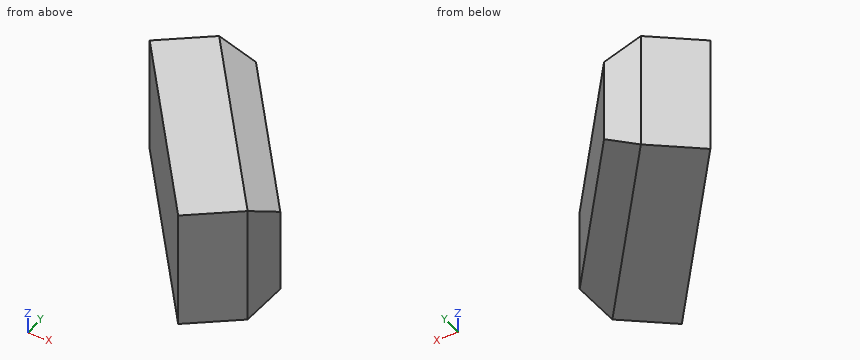
from build123d import *

# Parameters (mm, degrees)
SKETCH2_W             = 40
SKETCH2_H             = 80
BOSS_EXTRUDE1_DEPTH   = 30
CHAMFER1_SIZE         = 10
CHAMFER1_SIZE2        = 5.773502692
CHAMFER1_PART_2_SIZE  = 10
CHAMFER1_PART_2_SIZE2 = 5.773502692
CHAMFER1_PART_3_SIZE  = 10
CHAMFER1_PART_3_SIZE2 = 5.773502692
CHAMFER1_PART_4_SIZE  = 10
CHAMFER1_PART_4_SIZE2 = 5.773502692


with BuildPart() as part:
    # Sketch2 → Boss-Extrude1 (new body)
    with BuildSketch(Plane(origin=(0, 0, 0), x_dir=(0, 0, -1), z_dir=(0.788010754, 0.615661475, 0))):
        with Locations((20, 40)):
            Rectangle(SKETCH2_W, SKETCH2_H)
    extrude(amount=BOSS_EXTRUDE1_DEPTH)

    # Chamfer1
    chamfer1_edges = [part.edges().sort_by_distance(p)[0] for p in [
        (-0.986136405, 49.990274404, -40),
    ]]
    chamfer1_side = [part.faces().sort_by_distance(p)[0] for p in [
        (-12.806297709, 40.755352274, -40),
    ]]
    chamfer(chamfer1_edges, length=CHAMFER1_SIZE, length2=CHAMFER1_SIZE2, reference=chamfer1_side[0])

    # Chamfer1 part 2
    chamfer1_part_2_edges = [part.edges().sort_by_distance(p)[0] for p in [
        (-25.612595418, 81.510704548, -20),
    ]]
    chamfer1_part_2_side = [part.faces().sort_by_distance(p)[0] for p in [
        (-37.432756722, 72.275782418, -20),
    ]]
    chamfer(chamfer1_part_2_edges, length=CHAMFER1_PART_2_SIZE, length2=CHAMFER1_PART_2_SIZE2, reference=chamfer1_part_2_side[0])

    # Chamfer1 part 3
    chamfer1_part_3_edges = [part.edges().sort_by_distance(p)[0] for p in [
        (-0.986136405, 49.990274404, 0),
    ]]
    chamfer1_part_3_side = [part.faces().sort_by_distance(p)[0] for p in [
        (-12.806297709, 40.755352274, 0),
    ]]
    chamfer(chamfer1_part_3_edges, length=CHAMFER1_PART_3_SIZE, length2=CHAMFER1_PART_3_SIZE2, reference=chamfer1_part_3_side[0])

    # Chamfer1 part 4
    chamfer1_part_4_edges = [part.edges().sort_by_distance(p)[0] for p in [
        (23.640322608, 18.46984426, -20),
    ]]
    chamfer1_part_4_side = [part.faces().sort_by_distance(p)[0] for p in [
        (11.820161304, 9.23492213, -20),
    ]]
    chamfer(chamfer1_part_4_edges, length=CHAMFER1_PART_4_SIZE, length2=CHAMFER1_PART_4_SIZE2, reference=chamfer1_part_4_side[0])


solid = part.part
Verification items for the finished model (mm, model axes). Coordinates: 2 decimals unless noted, no trailing zeros. Order: outer loops, then holes, each group sorted by start corner. A loop starts at its lowest first (then second) coordinate and runs counter-clockwise, first axis right, second up.
1. Sectioned sample at A-A, the plane z = -13. Record the cut outline in (x, y).
Results found:
outline: (-49.25, 63.04) - (0, 0) - (15.76, 12.31) - (20.09, 23.02) - (-22.06, 76.96) - (-33.49, 75.35) - close
2. Sectioned sample at B-B, the plane x = 6.5. Record the cut outline in (y, z).
Results found:
outline: (5.08, -40) - (24.17, -40) - (40.41, -34.23) - (40.41, -5.77) - (24.17, 0) - (5.08, 0) - close
3. Sectioned sample at C-C, the plane y = 11. Record the cut outline in (x, z), and give its area (3 significant figures).
Results found:
outline: (-8.59, -40) - (14.08, -40) - (14.08, 0) - (-8.59, 0) - close
area: 907 mm2
4. Sectioned sample at D-D, the plane x = -39.5. Record the cut outline in (y, z).
Results found:
outline: (50.56, -40) - (70.66, -40) - (70.66, 0) - (50.56, 0) - close
5. Scan lines: line 1 (Y direction, x = -44.5, z = -10); line 2 (Y direction, x = -30, z = -15.5); line 3 (X direction, y = 22, z = -29.5). Record each from-to range of solid material in increasing order.
Results found:
line 1: y = 56.96 to 66.75
line 2: y = 38.4 to 75.84
line 3: x = -17.19 to 19.67
6. Go/stop test with flat-tipped pins: pin 1 Ø4 at (y, z) = (13, -7) entering from -X; pin 2 Ø5 at (y, z) = (15.5, -31.5) entering from -X; pin 3 Ø5 at (y, z) = (51.5, -32.5) entering from -X. Record where each tip stops, or that it passes through.
Results found:
pin 1: stops at x = -11.72
pin 2: stops at x = -14.06
pin 3: stops at x = -42.19
